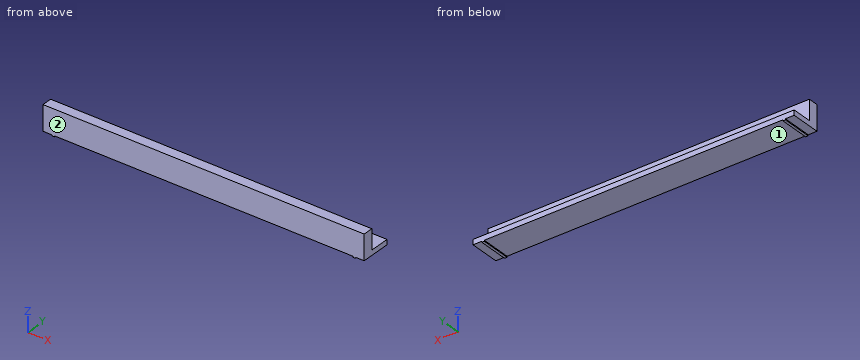
```python
from build123d import *

# Parameters (mm, degrees)
SKETCH1_W           = 812.8
SKETCH1_H           = 76.114888738
BOSS_EXTRUDE1_DEPTH = 12.7
BOSS_EXTRUDE2_DEPTH = 25.4
SKETCH3_W           = 6.35
SKETCH3_H           = 76.114888738
BOSS_EXTRUDE4_DEPTH = 2.54


with BuildPart() as part:
    # Sketch1 → Boss-Extrude1 (new body)
    with BuildSketch(Plane.XY):
        with Locations((406.4, 38.057444369)):
            Rectangle(SKETCH1_W, SKETCH1_H)
    extrude(amount=BOSS_EXTRUDE1_DEPTH)

    # Sketch2 → Boss-Extrude2 (add)
    with BuildSketch(Plane.XZ):
        Polygon((0, 12.7), (0, 63.5), (812.8, 63.5), (812.8, 12.7), (812.8, 0), (0, 0), align=None)
    extrude(amount=-BOSS_EXTRUDE2_DEPTH)

    # Sketch3 → Boss-Extrude4 (add)
    with BuildSketch(Plane(origin=(0, 0, 0), x_dir=(-1, 0, 0), z_dir=(0, 0, -1))):
        with Locations((-787.4, 38.057444369)):
            Rectangle(SKETCH3_W, SKETCH3_H)
        with Locations((-25.4, 38.057444369)):
            Rectangle(SKETCH3_W, SKETCH3_H)
    extrude(amount=BOSS_EXTRUDE4_DEPTH)


solid = part.part
```
Input: part model. Units: mm. Frame: model coordinates. Face numbers are marked on the shaded views. Give positions to 0.01 mm unless a question says otherwise; leave off trailing zeros. Write each loop counter-clockwise with the first axis right and the second up, starting at its lowest first coordinate (ties: lowest second). Pieces come first, ordered by that corner, then holes. Notation, with made-up numbers: (25, 8.5) - (35, 8.5) arc R23 cw to (35, 16.5) - close; hole circle Ø7 at (25.5, 73.5). An arc over 180 degrees is marked (long way). Write item = value, one per line. Start each with the question number.
1) Material intervals for L1, parallel to Z at x = 379, y = 60.5; L2, parallel to Z at x = 262, y = 9.5; L3, parallel to Y at x = 403, z = 56, sorted ascending. Write a range as [from, to].
2) Cut plane C-C (z = 53.5). Return loops of the section in (x, y).
3) Draft query along X for the marked faces 1 and 2. Return one class per face: pulls with the +X half, pulls with the -X half, needs draft (parallel to the pull), parting line crosses it, or undercut.
4) Cut plane D-D (y = 49). Return loops of the section in (x, z) (3 decimals).
5) Cut plane A-A (y = 11.5). Return loops of the section in (x, z) (3 decimals), and give its area (3 significant figures).
6) Pin query (flat end, axial travel): pin 1 (6 mm diameter, centred on x = 439, z = 52, fed in from +Y); pin 2 (3 mm diameter, centred on y = 30, z = -0.5, fed in from -X); pin 3 (12 mm diameter, centred on x = 146, y = 21.5, fed in from -Z); pin 4 (0.8 mm diameter, centred on y = 42.5, z = -1, fed in from -X) (3 decimals). Return the tip coordinate at first contact, or that it passes through.
7) Cut plane B-B (x = 114.5). Return loops of the section in (y, z), and give its area (3 significant figures).
Answers follow:
q1.L1 = [0, 12.7]
q1.L2 = [0, 63.5]
q1.L3 = [0, 25.4]
q2.outline = (0, 0) - (812.8, 0) - (812.8, 25.4) - (0, 25.4) - close
q3.face_1 = undercut
q3.face_2 = needs draft
q4.outline = (0, 0) - (22.225, 0) - (22.225, -2.54) - (28.575, -2.54) - (28.575, 0) - (784.225, 0) - (784.225, -2.54) - (790.575, -2.54) - (790.575, 0) - (812.8, 0) - (812.8, 12.7) - (0, 12.7) - close
q5.outline = (0, 0) - (22.225, 0) - (22.225, -2.54) - (28.575, -2.54) - (28.575, 0) - (784.225, 0) - (784.225, -2.54) - (790.575, -2.54) - (790.575, 0) - (812.8, 0) - (812.8, 63.5) - (0, 63.5) - close
q5.area = 51,600 mm^2
q6.pin_1 = 25.4
q6.pin_2 = 0
q6.pin_3 = 0
q6.pin_4 = 22.225
q7.outline = (0, 0) - (76.11, 0) - (76.11, 12.7) - (25.4, 12.7) - (25.4, 63.5) - (0, 63.5) - close
q7.area = 2,260 mm^2
